```python
from build123d import *

# Parameters (mm, degrees)
BOSS_EXTRUDE2_DEPTH   = 8
M4_TAPPED_HOLE1_D     = 3.3
M4_TAPPED_HOLE1_DEPTH = 11.5
M4_TAPPED_HOLE1_TIP   = 0.991420021
M3_TAPPED_HOLE1_D     = 2.5
M3_TAPPED_HOLE1_DEPTH = 8.5
M3_TAPPED_HOLE1_TIP   = 0.751075774


with BuildPart() as part:
    # Sketch1 → Boss-Extrude2 (new body)
    with BuildSketch(Plane(origin=(0, 0, 0), x_dir=(1, 0, 0), z_dir=(0, 1, 0))):
        Polygon((-35, -4), (-27, 4), (35, 4), (35, -4), (-6.5, -4), (-6.5, -9), (-14, -9), (-21.25, -1.75), (-28.5, -9), (-35, -9), align=None)
    extrude(amount=BOSS_EXTRUDE2_DEPTH)

    # M4 Tapped Hole1
    with Locations(Plane(origin=(0, 0, -4), x_dir=(-1, 0, 0), z_dir=(0, 0, -1))):
        with Locations((21.25, 4)):
            Hole(M4_TAPPED_HOLE1_D / 2, depth=M4_TAPPED_HOLE1_DEPTH)
            with Locations((0, 0, -(M4_TAPPED_HOLE1_DEPTH + M4_TAPPED_HOLE1_TIP / 2))):  # 118° drill point
                Cone(0, M4_TAPPED_HOLE1_D / 2, M4_TAPPED_HOLE1_TIP, mode=Mode.SUBTRACT)

    # M3 Tapped Hole1
    with Locations(Plane(origin=(0, 0, -4), x_dir=(-1, 0, 0), z_dir=(0, 0, -1))):
        with Locations((-31, 4), (-24, 4)):
            Hole(M3_TAPPED_HOLE1_D / 2, depth=M3_TAPPED_HOLE1_DEPTH)
            with Locations((0, 0, -(M3_TAPPED_HOLE1_DEPTH + M3_TAPPED_HOLE1_TIP / 2))):  # 118° drill point
                Cone(0, M3_TAPPED_HOLE1_D / 2, M3_TAPPED_HOLE1_TIP, mode=Mode.SUBTRACT)


solid = part.part
```
Input: part model. Units: mm. Frame: model coordinates. A direction names the side the tool comes from. Give positions to 0.01 mm unless a question says otherwise; leave off trailing zeros. Loops run counter-clockwise (first coordinate to the right, second up) from the corner with the lowest first, then second, coordinate; pieces in that order, holes last.
1) Reachability of faces 1 (the flat face through (-6.5, 4, 6)), 2 (the flat face through (-10, 4, 9)), 3 (the flat face through (-18, 4, 5)) from +Z, -Z, +X, -X, +Y, -Y: full face, straight path, thin tool, end or side. Return the list, or none.
A:
face 1: +Z, +X, +Y, -Y
face 2: +Z, +X, -X, +Y, -Y
face 3: +Z, +Y, -Y
2) Section query D-D on x = -22. Return the cut outline in (y, z), and give its area (3 significant figures).
A:
outline: (0, -4) - (2.53, -4) - (2.53, 2.5) - (0, 2.5) - close; (5.47, -4) - (8, -4) - (8, 2.5) - (5.47, 2.5) - close
area: 32.9 mm2
3) Section query A-A on y = 1.25. Return the cut outline in (x, z).
A:
outline: (-35, 4) - (-27, -4) - (35, -4) - (35, 4) - (-6.5, 4) - (-6.5, 9) - (-14, 9) - (-21.25, 1.75) - (-28.5, 9) - (-35, 9) - close
4) Section query B-B on x = 24. Return the cut outline in (y, z), and give its area (3 significant figures).
A:
outline: (0, -4) - (2.75, -4) - (2.75, 4) - (0, 4) - close; (5.25, -4) - (8, -4) - (8, 4) - (5.25, 4) - close
area: 44.0 mm2
5) Line query: L1, parallel to Y at x = 24, z = 0.75; L2, parallel to X at y = 3.5, z = 2.25; L3, parallel to Y at x = -21.25, z = 0.5. Output: solid intervals per line, ascending.
A:
L1: y = 0 to 2.75, 5.25 to 8
L2: x = -33.25 to -22.82, -19.68 to 22.85, 25.15 to 29.85, 32.15 to 35
L3: y = 0 to 2.35, 5.65 to 8
6) Contact query for flat-ended pins moving along their axis: pin 1 (3 mm diameter, centred on x = -21.25, y = 4, fed in from +Z); pin 2 (2.5 mm diameter, centred on x = 21.5, y = 3.5, fed in from +Z); pin 3 (4 mm diameter, centred on y = 6, z = 1.5, fed in from -X); pin 4 (4 mm diameter, centred on y = 4, z = 6.5, fed in from +X). Output: stop coordinate, or through.
A:
pin 1: passes through
pin 2: stops at z = 4
pin 3: stops at x = -34.5
pin 4: stops at x = -6.5
7) Section query C-C on z = -1.5. Return the cut outline in (x, y), and give its area (3 significant figures).
A:
outline: (-29.5, 0) - (35, 0) - (35, 8) - (-29.5, 8) - close; hole circle Ø3.3 at (-21.25, 4); hole circle Ø2.5 at (24, 4); hole circle Ø2.5 at (31, 4)
area: 498 mm2
8) Mould query, pull axis Y, two halves, no side actions, for faces 4 (the flat face through (0, 8, 1)), 5 (the cylindrical face through (-20.489, 2.536, -0.248)), 6 (the flat face through (-32, 4, 9)). Classes: released by +Y, released by -Y, zero draft, split by the parting line, or undercut.
A:
face 4: released by +Y
face 5: undercut
face 6: zero draft
